Geometry check sheet. Reference: the model listing, model coordinates, mm. Round coordinates to 2 decimals unless told otherwise and drop trailing zeros. Order: outer loops, then holes, each group sorted by start corner. A loop starts at its lowest first (then second) coordinate and runs counter-clockwise, first axis right, second up. Notation, with made-up numbers: (-6.75, 15.5) -> (34.25, 15.5) arc R21 ccw to (34.25, 35.5) -> close; hole circle Ø11 at (74.5, 3.5). An arc over 180 degrees is marked (long way). Use a Markdown table: item, result. Add a question column.
Item 1: Sectioned sample at A-A, the plane y = 0. Record the cut outline in (x, z) (3 decimals), and give its area (3 significant figures).
Item 2: Gauge pin test, flat ends, axial feed: pin 1 Ø4.5 at (x, y) = (0, 0) entering from +Z; pin 2 Ø1 at (x, z) = (-7, 1) entering from -Y; pin 3 Ø1.6 at (x, z) = (-23, 1.5) entering from +Y. Record the tip position at first contact, or that the pin passes through.
Item 3: Sectioned sample at D-D, the plane y = -14. Record the cut outline in (x, z) (3 decimals).
Item 4: Sectioned sample at B-B, the plane z = 2.55. Record the cut outline in (x, y).
Item 5: Material ranges on probe 1 along Y at (x, z) = (0, 1.2); probe 2 along X at (y, z) = (-39.5, 1.4); probe 3 along Y at (x, z) = (-12.5, 0.7), recorded low to high. Write a range as [from, to].
Item 6: Sectioned sample at C-C, the plane x = -25. Record the cut outline in (y, z) (3 decimals), and give its area (3 significant figures).
from build123d import *

# Parameters (mm, degrees)
BOSS_EXTRUDE1_DEPTH = 3.175
FILLET1_R           = 7
FILLET2_R           = 5
SKETCH2_R           = 2.38125
CUT_EXTRUDE1_DEPTH  = 62.693440697
LPATTERN1_COUNT     = 3
LPATTERN1_PITCH     = 12.5


with BuildPart() as part:
    # Sketch1 → Boss-Extrude1 (new body)
    with BuildSketch(Plane.XY):
        with BuildLine():
            Line((-11.618950039, 11), (-36, 11))
            Line((-36, 11), (-36, -39))
            ThreePointArc((-36, -39), (-25, -50), (-14, -39))
            Line((-14, -39), (-14, -11))
            Line((-14, -11), (-11.618950039, -11))
            ThreePointArc((-11.618950039, -11), (16, 0), (-11.618950039, 11))
        make_face()
    extrude(amount=BOSS_EXTRUDE1_DEPTH)

    # Fillet1
    fillet1_edges = [part.edges().sort_by_distance(p)[0] for p in [
        (-36, 11, 1.5875),
    ]]
    fillet(fillet1_edges, radius=FILLET1_R)

    # Fillet2
    # the kernel refuses this fillet: 5 mm, written as the material it adds along each edge
    with BuildSketch(Plane(origin=(-14, -11, 0), x_dir=(1, 0, 0), z_dir=(0, 0, 1))) as fillet2_piece_1:
        with BuildLine():
            CenterArc((5, -4.259237102), FILLET2_R, 121.586822832, 58.413177168)
            Line((0, -4.259237102), (-0.1, -4.259237102))
            Line((-0.1, -4.259237102), (-0.1, 0))
            Line((-0.1, 0), (0, 0.1))
            ThreePointArc((0, 0.1), (1.190524981, 0.1), (2.328670961, 0.085184742))
            Line((2.328670961, 0.085184742), (2.381049961, 0))
        make_face()
    extrude(amount=3.175)

    # Sketch2 → Cut-Extrude1 (cut, through all)
    with BuildSketch(Plane.XY.offset(3.175)):
        Circle(SKETCH2_R)
    cut_extrude1 = extrude(amount=-CUT_EXTRUDE1_DEPTH, mode=Mode.SUBTRACT)

    # LPattern1: Cut-Extrude1 ×3
    with Locations(*[(-i * LPATTERN1_PITCH, 0, 0) for i in range(1, LPATTERN1_COUNT)]):
        add(cut_extrude1, mode=Mode.SUBTRACT)


solid = part.part
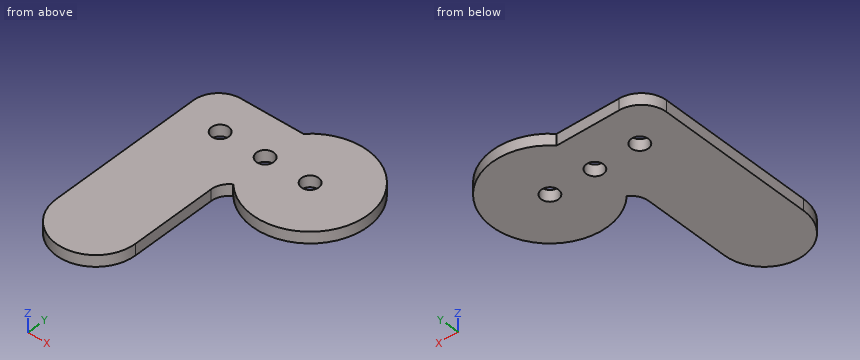
Found:
| question | item | result |
|---|---|---|
| 1 | outline | (-36, 0) -> (-27.381, 0) -> (-27.381, 3.175) -> (-36, 3.175) -> close; (-22.619, 0) -> (-14.881, 0) -> (-14.881, 3.175) -> (-22.619, 3.175) -> close; (-10.119, 0) -> (-2.381, 0) -> (-2.381, 3.175) -> (-10.119, 3.175) -> close; (2.381, 0) -> (16, 0) -> (16, 3.175) -> (2.381, 3.175) -> close |
| 1 | area | 120 mm2 |
| 2 | pin 1 | passes through |
| 2 | pin 2 | stops at y = -14.62 |
| 2 | pin 3 | stops at y = 11 |
| 3 | outline | (-36, 0) -> (-13.839, 0) -> (-13.839, 3.175) -> (-36, 3.175) -> close; (-7.746, 0) -> (7.746, 0) -> (7.746, 3.175) -> (-7.746, 3.175) -> close |
| 4 | outline | (-36, -39) arc R11 ccw to (-14, -39) -> (-14, -15.26) arc R5 cw to (-11.62, -11) arc R16 ccw (long way) to (-11.62, 11) -> (-29, 11) arc R7 ccw to (-36, 4) -> close; hole circle Ø4.76 at (-25, 0); hole circle Ø4.76 at (-12.5, 0); hole circle Ø4.76 at (0, 0) |
| 5 | probe 1 | y = [-16, -2.38], [2.38, 16] |
| 5 | probe 2 | x = [-35.99, -14.01] |
| 5 | probe 3 | y = [-11.69, -2.38], [2.38, 11] |
| 6 | outline | (-50, 0) -> (-2.381, 0) -> (-2.381, 3.175) -> (-50, 3.175) -> close; (2.381, 0) -> (11, 0) -> (11, 3.175) -> (2.381, 3.175) -> close |
| 6 | area | 179 mm2 |
